Autodesk Fusion 360 part; units mm, degrees
sketch "Sketch1" plane through (0, 0, 0) normal (0, 1, 0) x (1, 0, 0)
  line L0 (0, 0) -> (89.803, 0)
  line L1 (89.803, 0) -> (89.803, 89.803)
  line L2 (89.803, 89.803) -> (0, 89.803)
  line L3 (0, 89.803) -> (0, 0)
  dimension "d1" = 89.803
  dimension "d2" = 89.803
extrude "Extrude1" add sketch "Sketch1" along normal blind 10 makes body 1
sketch "Sketch6" plane through (0, 0, 0) normal (0, -1, 0) x (1, 0, 0)
  line L0 (0, -89.803) -> (89.803, -89.803)
  line L1 (89.803, -89.803) -> (89.803, 0)
  line L2 (89.803, 0) -> (0, 0)
  line L3 (77.4015, -12.4015) -> (12.4015, -12.4015)
  line L4 (12.4015, -12.4015) -> (12.4015, -77.4015)
  line L5 (12.4015, -77.4015) -> (77.4015, -77.4015)
  line L6 (77.4015, -77.4015) -> (77.4015, -12.4015)
  line L7 (77.4015, -12.4015) -> (12.4015, -77.4015) construction
  line L8 (12.4015, -12.4015) -> (77.4015, -77.4015) construction
  point P0 (44.9015, -44.9015)
  dimension "d12" = 65
  dimension "d13" = 65
extrude "Extrude3" add sketch "Sketch6" against normal blind 1 bodies 1
fillet "Fillet2" radius 3 8 edges at (0, 5, 0) (44.9015, 10, 0) (0, 10, -44.9015) (89.803, 10, -44.9015) (44.9015, 10, -89.803) (89.803, 5, 0) (89.803, 5, -89.803) (0, 5, -89.803) on bodies 1
copy_body "Body->Comp2" bodies 1 removing the originals makes body 2 in component "topbody2"
sketch "Sketch7" plane through (0, 0, 0) normal (0, -1, 0) x (1, 0, 0)
  arc A0 (86.803, -89.803) -> (89.803, -86.803) centre (86.803, -86.803) ccw
  line L0 (89.803, -86.803) -> (89.803, -3)
  arc A1 (89.803, -3) -> (86.803, 0) centre (86.803, -3) ccw
  line L1 (86.803, 0) -> (3, 0)
  arc A2 (3, 0) -> (0, -3) centre (3, -3) ccw
  line L2 (0, -3) -> (0, -86.803)
  arc A3 (0, -86.803) -> (3, -89.803) centre (3, -86.803) ccw
  line L3 (3, -89.803) -> (86.803, -89.803)
  circle A4 centre (5, -5) radius 3
  circle A5 centre (5, -85) radius 3
  circle A6 centre (85, -85) radius 3
  circle A7 centre (85, -5) radius 3
  dimension "d17" = 6
  dimension "d18" = 6
  dimension "d19" = 6
  dimension "d20" = 6
extrude "Extrude1'" cut sketch "Sketch7" against normal blind 3 contours A4 | A5 | A6 | A7 bodies 2 in component "topbody2"
sketch "Sketch8" plane through (0, 0, 0) normal (0, -1, 0) x (1, 0, 0)
  circle A0 centre (85, -5) radius 3
  circle A1 centre (85, -85) radius 3
  circle A2 centre (5, -5) radius 3
  circle A3 centre (5, -85) radius 3
  arc A4 (86.803, -89.803) -> (89.803, -86.803) centre (86.803, -86.803) ccw
  line L0 (89.803, -86.803) -> (89.803, -3)
  arc A5 (89.803, -3) -> (86.803, 0) centre (86.803, -3) ccw
  line L1 (86.803, 0) -> (3, 0)
  arc A6 (3, 0) -> (0, -3) centre (3, -3) ccw
  line L2 (0, -3) -> (0, -86.803)
  arc A7 (0, -86.803) -> (3, -89.803) centre (3, -86.803) ccw
  line L3 (3, -89.803) -> (86.803, -89.803)
  line L4 (7.6, -15) -> (7.6, -75)
  line L5 (14.4179, -82.203) -> (69.8225, -82.203)
  line L6 (82.203, -71.2718) -> (82.203, -12.7891)
  line L7 (70, -7.6) -> (20, -7.6)
  line L8 (7.6, -15) -> (7.6, -7.6)
  line L9 (7.6, -7.6) -> (20, -7.6)
  line L10 (7.6, -7.6) -> (20, -7.6)
  line L11 (20, -7.6) -> (70, -7.6)
  line L12 (70, -7.6) -> (82.203, -7.6)
  line L13 (82.203, -12.7891) -> (82.203, -7.6)
  line L14 (82.203, -71.2718) -> (82.203, -82.203)
  line L15 (69.8225, -82.203) -> (82.203, -82.203)
  line L16 (14.4179, -82.203) -> (7.6, -82.203)
  line L17 (7.6, -75) -> (7.6, -82.203)
extrude "Extrude2" add sketch "Sketch8" along normal blind 5 contours L4 L5 L6 L7 L8 L9 L10 L11 L12 L13 L14 L15 L16 L17 bodies 2 in component "topbody2"
sketch "Sketch9" plane through (0, -5, 0) normal (0, -1, 0) x (1, 0, 0)
  line L0 (7.6, -7.6) -> (7.6, -82.203)
  line L1 (7.6, -82.203) -> (82.203, -82.203)
  line L2 (82.203, -82.203) -> (82.203, -7.6)
  line L3 (82.203, -7.6) -> (7.6, -7.6)
  line L4 (78.6515, -11.1515) -> (11.1515, -11.1515)
  line L5 (11.1515, -11.1515) -> (11.1515, -78.6515)
  line L6 (11.1515, -78.6515) -> (78.6515, -78.6515)
  line L7 (78.6515, -78.6515) -> (78.6515, -11.1515)
  line L8 (78.6515, -11.1515) -> (11.1515, -78.6515) construction
  line L9 (11.1515, -11.1515) -> (78.6515, -78.6515) construction
  point P0 (44.9015, -44.9015)
  dimension "d33" = 67.5
  dimension "d34" = 67.5
extrude "Extrude3'" cut sketch "Sketch9" against normal blind 10 contours L4 L5 L6 L7 bodies 2 in component "topbody2"
component "topbody2" placed x (1, 0, 0) y (0, 1, 0) z (0, 0, 1) at (0, 0, 0)
Work out the finished part from the listing and answer in its coordinate system (mm). A direction names the side the tool comes from. Give positions to 0.01 mm unless a question says otherwise; leave off trailing zeros. Order: outer loops, then holes, each group sorted by start corner. A loop starts at its lowest first (then second) coordinate and runs counter-clockwise, first axis right, second up.
1. The mould has two halves that part along Z. Classify faces 4 (the flat face through (44, 5, -44)), 5 (the flat face through (78.652, 0, -45)), 6 (the flat face through (45, 3, -89.803)), 7 (the flat face through (44, -2, -7.6)): released by +Z, released by -Z, zero draft, split by the parting line, or undercut.
Result sheet:
face 4: undercut
face 5: undercut
face 6: released by -Z
face 7: released by +Z
2. Section A-A, the plane z = -85 is taken. Determine the outline of the cut face in (x, y).
Result sheet:
outline: (0, 0) - (2, 0) - (2, 3) - (8, 3) - (8, 0) - (82, 0) - (82, 3) - (88, 3) - (88, 0) - (89.8, 0) - (89.8, 7) arc R3 ccw to (86.8, 10) - (3, 10) arc R3 ccw to (0, 7) - close
3. For faces 1 (the cylindrical face through (82, 1, -5)), 2 (the flat face through (44, -2, -82.203)), 3 (the flat face through (0, 3, -45)), determine the directions among +Z, -Z, +X, -X, +Y, -Y from which every point of the face is accessible in a straight line to the end or side of a thin tool.
Result sheet:
face 1: -Y
face 2: -Z, +X, -X, -Y
face 3: +Z, -Z, -X, +Y, -Y
4. Section B-B, the plane x = 5 is taken. Determine the outline of the cut face in (y, z).
Result sheet:
outline: (0, -89.8) - (7, -89.8) arc R3 ccw to (10, -86.8) - (10, -3) arc R3 ccw to (7, 0) - (0, 0) - (0, -2) - (3, -2) - (3, -8) - (0, -8) - (0, -82) - (3, -82) - (3, -88) - (0, -88) - close
5. Straight lines are drawn through the part: L1, parallel to Z at x = 85, y = 0.7; L2, parallel to X at y = -2, z = -61; L3, parallel to X at y = 1, z = -51. For each, find the intervals that lie inside material, in ascending order.
Result sheet:
L1: z = -89.8 to -88, -82 to -8, -2 to 0
L2: x = 7.6 to 11.15, 78.65 to 82.2
L3: x = 0 to 11.15, 78.65 to 89.8
6. Each of these flat-tipped pins is pushed along its axis until it touches: P1, Ø7, axis at x = 5, z = -5, coming from the -Y side; P2, Ø1.8, axis at x = 85.5, z = -85.5, coming from the -Y side; P3, Ø5.5, axis at y = -3.5, z = -29, coming from the -X side. Where does it stop, or does it pass through?
Result sheet:
P1: stops at y = 0
P2: stops at y = 3
P3: stops at x = 7.6
